Part print with two shaded views. Sizes in mm from the minimum x, y, z corner. A direction names the side the tool comes from. Give positions to 0.01 mm unless a question says otherwise; leave off trailing zeros. Write each loop counter-clockwise with the first axis right and the second up, starting at its lowest first coordinate (ties: lowest second). Pieces come first, ordered by that corner, then holes.
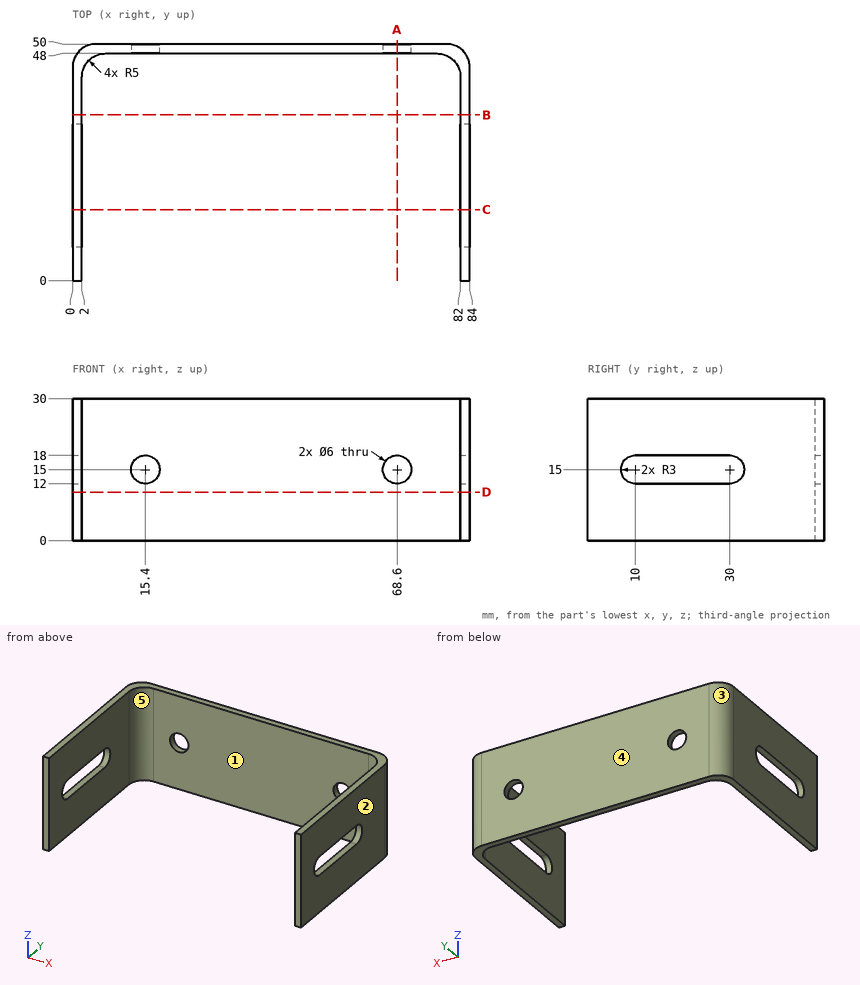
1) Saw through at A-A, the plane x = 68.6. Write the cut outline in (y, z).
Answers follow:
outline: (48, 0) - (50, 0) - (50, 12) - (48, 12) - close; (48, 18) - (50, 18) - (50, 30) - (48, 30) - close
2) 3-axis set-ups, long thin cutter, end or side, ignore diameter. For the marked faces 1 and 2: which of +Z, -Z, +X, -X, +Y, -Y reach the whole face in a straight line?
Answers follow:
face 1: +Z, -Z, -Y
face 2: +Z, -Z, +X, +Y, -Y
3) Saw through at C-C, the plane y = 15. Write the cut outline in (x, z).
Answers follow:
outline: (0, 0) - (2, 0) - (2, 12) - (0, 12) - close; (0, 18) - (2, 18) - (2, 30) - (0, 30) - close; (82, 0) - (84, 0) - (84, 12) - (82, 12) - close; (82, 18) - (84, 18) - (84, 30) - (82, 30) - close
4) Wall check: L1, parallel to Z at x = 15.4, y = 49.1; L2, parallel to X at y = 39.5, z = 23.25; L3, parallel to Y at x = 61, z = 6. Give the ranges that are in metal, low to high.
Answers follow:
L1: z = 0 to 12, 18 to 30
L2: x = 0 to 2, 82 to 84
L3: y = 48 to 50
5) Two-plate mould, pull along X, no slides. Class the marked faces 3, 4 and 5: +X half, -X half, draft (parallel to the pull), parting line (faces both ways), or undercut.
Answers follow:
face 3: -X half
face 4: draft
face 5: undercut
6) Pin check, flat tips, straight feed: pin 1 Ø2 at (x, z) = (39.5, 4) entering from -Y; pin 2 Ø6 at (x, z) = (17.5, 16.5) entering from +Y. Stop position of each tip, or through.
Answers follow:
pin 1: stops at y = 48
pin 2: stops at y = 50
7) Saw through at B-B, the plane y = 35. Write the cut outline in (x, z), then the cut area to 3 significant figures.
Answers follow:
outline: (0, 0) - (2, 0) - (2, 30) - (0, 30) - close; (82, 0) - (84, 0) - (84, 30) - (82, 30) - close
area: 120 mm2
8) Saw through at D-D, the plane z = 10.25. Write the cut outline in (x, y).
Answers follow:
outline: (0, 0) - (2, 0) - (2, 43) arc R5 cw to (7, 48) - (77, 48) arc R5 cw to (82, 43) - (82, 0) - (84, 0) - (84, 45) arc R5 ccw to (79, 50) - (5, 50) arc R5 ccw to (0, 45) - close
